Geometry check sheet. Reference: the model listing, model coordinates, mm. Face numbers are marked on the shaded views. A direction names the side the tool comes from. Round coordinates to 2 decimals unless told otherwise and drop trailing zeros. Order: outer loops, then holes, each group sorted by start corner. A loop starts at its lowest first (then second) coordinate and runs counter-clockwise, first axis right, second up.
(1) Cross-section at B-B on z = 0. Enter the section's corners in (x, y), and give its area (3 significant figures).
(2) Cross-section at D-D on x = 1.75. Enter the section's corners in (y, z), and give its area (3 significant figures).
(3) Cross-section at C-C on y = 19.75. Enter the section's corners in (x, z).
(4) Set-up check for the marked faces 1 and 2: record each of +Z, -Z, +X, -X, +Y, -Y from which the full face is reachable in a straight line by a thin tool's end or side.
(5) Thickness scan on L1, parallel to Z at x = 0, y = 22.85; L2, parallel to Y at x = 2.5, z = 0.75. Record the ranges inside material, lowest first.
(6) Draft check along X on the marked faces 3, 4 and 5. Enter one of: pulls with the +X half, pulls with the -X half, needs draft (parallel to the pull), parting line crosses it, or undercut.
(7) Gauge pin test, flat ends, axial feed: P1, Ø1.5, axis at x = 0, y = 17.5, coming from the +Z side; P2, Ø0.9, axis at x = 0.5, z = -0.5, coming from the +Y side. Record the tip position at first contact, or that the pin passes through.
(8) Cross-section at A-A on x = 0. Enter the section's corners in (y, z).
from build123d import *

# Parameters (mm, degrees)
SKETCH1_R           = 2.5
BOSS_EXTRUDE1_DEPTH = 20
SKETCH2_R           = 4
BOSS_EXTRUDE2_DEPTH = 5
SKETCH3_R           = 1.5
CUT_EXTRUDE1_DEPTH  = 3


with BuildPart() as part:
    # Sketch1 → Boss-Extrude1 (new body)
    with BuildSketch(Plane(origin=(0, 0, 0), x_dir=(1, 0, 0), z_dir=(0, 1, 0))):
        Circle(SKETCH1_R)
    extrude(amount=BOSS_EXTRUDE1_DEPTH)

    # Sketch2 → Boss-Extrude2 (add)
    with BuildSketch(Plane(origin=(0, 20, 0), x_dir=(1, 0, 0), z_dir=(0, 1, 0))):
        Circle(SKETCH2_R)
    extrude(amount=BOSS_EXTRUDE2_DEPTH)

    # Sketch3 → Cut-Extrude1 (cut)
    with BuildSketch(Plane(origin=(0, 25, 0), x_dir=(1, 0, 0), z_dir=(0, 1, 0))):
        Circle(SKETCH3_R)
    extrude(amount=-CUT_EXTRUDE1_DEPTH, mode=Mode.SUBTRACT)


solid = part.part
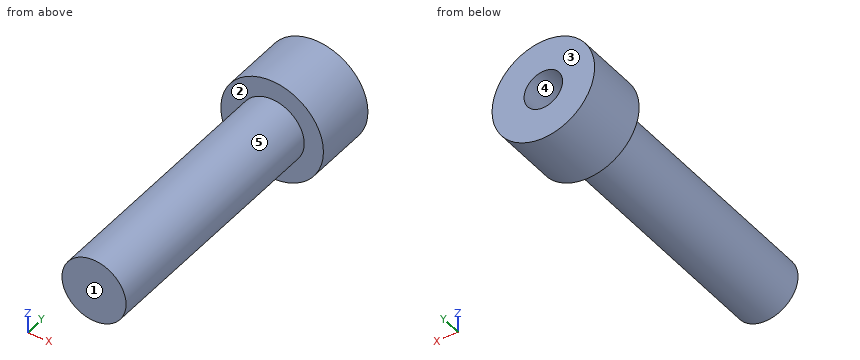
Found:
1. outline: (-4, 20) - (-2.5, 20) - (-2.5, 0) - (2.5, 0) - (2.5, 20) - (4, 20) - (4, 25) - (1.5, 25) - (1.5, 22) - (-1.5, 22) - (-1.5, 25) - (-4, 25) - close
1. area: 131 mm2
2. outline: (0, -1.79) - (20, -1.79) - (20, -3.6) - (25, -3.6) - (25, 3.6) - (20, 3.6) - (20, 1.79) - (0, 1.79) - close
2. area: 107 mm2
3. outline: circle Ø5 at (0, 0)
4. face 1: +Z, -Z, +X, -X, -Y
4. face 2: -Y
5. L1: z = -4 to -1.5, 1.5 to 4
5. L2: y = 20 to 25
6. face 3: needs draft
6. face 4: undercut
6. face 5: parting line crosses it
7. P1: stops at z = 2.5
7. P2: stops at y = 22
8. outline: (0, -2.5) - (20, -2.5) - (20, -4) - (25, -4) - (25, -1.5) - (22, -1.5) - (22, 1.5) - (25, 1.5) - (25, 4) - (20, 4) - (20, 2.5) - (0, 2.5) - close
